Design review of the part built by this model. Coordinates are the model's own, in mm. Coordinates: 2 decimals unless noted, no trailing zeros. Loops run counter-clockwise (first coordinate to the right, second up) from the corner with the lowest first, then second, coordinate; pieces in that order, holes last. Notation, with made-up numbers: (39, -15.75) -> (46, -15.75) arc R9 ccw to (46, 1.25) -> close; hole circle Ø2 at (33, 37.25). An arc over 180 degrees is marked (long way). Use one line per item in the form item = value. Start each with the question number.
1. For pin 1 (1.3 mm diameter, centred on x = 100.5, z = 40, fed in from -Y); pin 2 (1 mm diameter, centred on x = 21, y = 2.5, fed in from -Z); pin 3 (12 mm diameter, centred on y = 18.5, z = 20, fed in from -X) (3 decimals), all flat-tipped, find the tip position at first contact; note any pin that passes through.
2. Wall thickness on line 1 (Y direction, x = 55, z = 1); line 2 (Y direction, x = 62, z = 2); line 3 (Z direction, x = 83, y = -1.5): over which ranges is each line inside the solid? List them lowest first. Write a range as from..to.
3. Consider section D-D (y = 11). State the section outline as (x, z) points (3 decimals), then the cut area to 3 significant figures.
4. Consider section A-A (z = 12.5). State the section outline as (x, y) points (3 decimals), then the cut area to 3 significant figures.
5. Consider section B-B (y = 1.25). State the section outline as (x, z) points (3 decimals), then the cut area to 3 significant figures.
6. Consider section C-C (z = 5). State the section outline as (x, y) points (3 decimals).
Autodesk Inventor part; units mm, degrees
ref_plane "Work Plane1" through (31.75, 0, 0) normal (1, 0, 0) x (0, 0, -1)
ref_plane "YZ Plane" through (0, 0, 0) normal (1, 0, 0) x (0, 1, 0)
ref_plane "XZ Plane" through (0, 0, 0) normal (0, 1, 0) x (-1, 0, 0)
sketch "Sketch1" plane through (0, 0, 0) normal (1, 0, 0) x (0, 1, 0)
  circle A0 centre (0, 0) radius 6.35
  dimension "d0" = 12.7
extrude "Extrusion1" add sketch "Sketch1" along normal blind 101.6
sketch "Sketch2" plane through (101.6, 0, 0) normal (1, 0, 0) x (0, 0, -1)
  line L0 (0, 0) -> (2.54, 0)
  line L1 (-40.64, 0) -> (-38.1, 0)
  arc A0 (0, 0) -> (-38.1, 0) centre (-19.05, 0) ccw
  arc A1 (2.54, 0) -> (-40.64, 0) centre (-19.05, 0) ccw
  dimension "d3" = 2.54
  dimension "d4" = 2.54
  dimension "d5" = 38.1
  dimension "d6" = 19.05
extrude "Extrusion2" add sketch "Sketch2" against normal blind 3.175
ref_plane "Work Plane1" through (31.75, 0, 0) normal (1, 0, 0) x (0, 0, -1)
sketch "Sketch3" plane through (31.75, 0, 0) normal (1, 0, 0) x (0, 0, -1)
  line L0 (0, 0) -> (2.54, 0)
  line L1 (-38.1, 0) -> (-40.64, 0)
  arc A0 (0, 0) -> (-38.1, 0) centre (-19.05, 0) ccw
  arc A1 (-1.0583, 6.2612) -> (-38.1, 0) centre (-19.05, 0) ccw
  line L2 (-1.0583, 6.2612) -> (0, 0)
  arc A2 (2.54, 0) -> (-40.64, 0) centre (-19.05, 0) ccw
  line L3 (-38.1, 0) -> (-40.64, 0) construction
  line L4 (0, 0) -> (2.54, 0) construction
  arc A3 (1.651, 6.1316) -> (-40.64, 0) centre (-19.05, 0) ccw
  arc A4 (1.651, 6.1316) -> (-1.0583, 6.2612) centre (0, 0) ccw
  point P0 (0, 0)
  dimension "d10" = 2.54
  dimension "d11" = 2.54
  dimension "d12" = 38.1
  dimension "d13" = 19.05
  dimension "d14" = 180
  dimension "d15" = 6.35
extrude "Extrusion3" add sketch "Sketch3" against normal blind 3.175 contours A0 L1 A2 A4
properties part number "pincherRight"
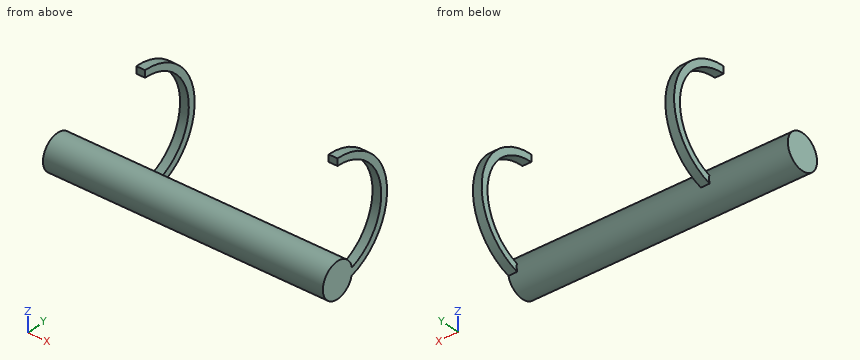
Geometry check:
q1.pin_1 = 0
q1.pin_2 = -6.03
q1.pin_3 = 28.575
q2.line_1 = -6.27..6.27
q2.line_2 = -6.03..6.03
q2.line_3 = -6.17..6.17
q3.outline = (28.575, 0.472) -> (31.75, 0.472) -> (31.75, 3.497) -> (28.575, 3.497) -> close; (28.575, 34.603) -> (31.75, 34.603) -> (31.75, 37.628) -> (28.575, 37.628) -> close; (98.425, 0.472) -> (101.6, 0.472) -> (101.6, 3.497) -> (98.425, 3.497) -> close; (98.425, 34.603) -> (101.6, 34.603) -> (101.6, 37.628) -> (98.425, 37.628) -> close
q3.area = 38.4 mm²
q4.outline = (28.575, 17.889) -> (31.75, 17.889) -> (31.75, 20.572) -> (28.575, 20.572) -> close; (98.425, 17.889) -> (101.6, 17.889) -> (101.6, 20.572) -> (98.425, 20.572) -> close
q4.area = 17.0 mm²
q5.outline = (0, -6.226) -> (101.6, -6.226) -> (101.6, 6.226) -> (0, 6.226) -> close; (28.575, 38.059) -> (31.75, 38.059) -> (31.75, 40.604) -> (28.575, 40.604) -> close; (98.425, 38.059) -> (101.6, 38.059) -> (101.6, 40.604) -> (98.425, 40.604) -> close
q5.area = 1,280 mm²
q6.outline = (0, -3.914) -> (101.6, -3.914) -> (101.6, 3.914) -> (0, 3.914) -> close; (28.575, 12.865) -> (31.75, 12.865) -> (31.75, 16.393) -> (28.575, 16.393) -> close; (98.425, 12.865) -> (101.6, 12.865) -> (101.6, 16.393) -> (98.425, 16.393) -> close
